```python
from build123d import *

# Parameters (mm, degrees)
SKETCH1_W                  = 480
SKETCH1_H                  = 70
SKETCH1_R                  = 19.15
SKETCH1_R_2                = 2.1
SKETCH1_R_3                = 7.1
BOSS_EXTRUDE1_DEPTH        = 10
M5_TAPPED_HOLE1_D          = 4.2
M5_TAPPED_HOLE1_DEPTH      = 12.4
M5_TAPPED_HOLE1_TIP        = 1.2618073
M5_TAPPED_HOLE2_D          = 4.2
M5_TAPPED_HOLE2_DEPTH      = 12.4
M5_TAPPED_HOLE2_TIP        = 1.2618073
F_3_3_3_3_DIAMETER_HOLE1_D = 3.3


with BuildPart() as part:
    # Sketch1 → Boss-Extrude1 (new body)
    with BuildSketch(Plane.XY):
        Rectangle(SKETCH1_W, SKETCH1_H)
        with Locations((0, -1)):
            Circle(SKETCH1_R, mode=Mode.SUBTRACT)
        with Locations((-23.55, -24.55)):
            Circle(SKETCH1_R_2, mode=Mode.SUBTRACT)
        with Locations((23.55, -24.55)):
            Circle(SKETCH1_R_2, mode=Mode.SUBTRACT)
        with Locations((23.55, 22.55)):
            Circle(SKETCH1_R_2, mode=Mode.SUBTRACT)
        with Locations((-23.55, 22.55)):
            Circle(SKETCH1_R_2, mode=Mode.SUBTRACT)
        with Locations((-215, -5)):
            Circle(SKETCH1_R_3, mode=Mode.SUBTRACT)
        with Locations((215, -5)):
            Circle(SKETCH1_R_3, mode=Mode.SUBTRACT)
    extrude(amount=BOSS_EXTRUDE1_DEPTH)

    # M5 Tapped Hole1
    with Locations(Plane(origin=(0, 35, 0), x_dir=(1, 0, 0), z_dir=(0, 1, 0))):
        with Locations((220, -5), (-220, -5), (-20, -5), (20, -5)):
            Hole(M5_TAPPED_HOLE1_D / 2, depth=M5_TAPPED_HOLE1_DEPTH)
            with Locations((0, 0, -(M5_TAPPED_HOLE1_DEPTH + M5_TAPPED_HOLE1_TIP / 2))):  # 118° drill point
                Cone(0, M5_TAPPED_HOLE1_D / 2, M5_TAPPED_HOLE1_TIP, mode=Mode.SUBTRACT)

    # M5 Tapped Hole2
    with Locations(Plane(origin=(0, -35, 0), x_dir=(-1, 0, 0), z_dir=(0, -1, 0))):
        with Locations((-220, -5), (220, -5)):
            Hole(M5_TAPPED_HOLE2_D / 2, depth=M5_TAPPED_HOLE2_DEPTH)
            with Locations((0, 0, -(M5_TAPPED_HOLE2_DEPTH + M5_TAPPED_HOLE2_TIP / 2))):  # 118° drill point
                Cone(0, M5_TAPPED_HOLE2_D / 2, M5_TAPPED_HOLE2_TIP, mode=Mode.SUBTRACT)

    # Ø3.3 (3.3) Diameter Hole1 (through all)
    with Locations(Plane.XY.offset(10)):
        with Locations((-200, 23), (-120, 23), (-40, 23), (40, 23), (120, 23), (200, 23)):
            Hole(F_3_3_3_3_DIAMETER_HOLE1_D / 2)


solid = part.part
```
Model file for the job. Use its own axes, mm. Round coordinates to 2 decimals unless told otherwise and drop trailing zeros. Order: outer loops, then holes, each group sorted by start corner. A loop starts at its lowest first (then second) coordinate and runs counter-clockwise, first axis right, second up. Notation, with made-up numbers: (20.5, 76.25) -> (25.5, 76.25) arc R33 ccw to (25.5, 111.25) -> close; hole circle Ø2 at (78.5, -4). An arc over 180 degrees is marked (long way). Use one line per item in the form item = value.
Item 1: Drill centre lines: line 1 (Y direction, x = -23.5, z = 6.5); line 2 (Y direction, x = -200, z = 3.75); line 3 (Z direction, x = -20, y = 30.75). Where is each one in solid material? Low to high.
Returned:
line_1 = -35 to -26.65, -22.45 to 20.45, 24.65 to 35
line_2 = -35 to 21.35, 24.65 to 35
line_3 = 0 to 2.9, 7.1 to 10
Item 2: Flat gauge pins, fed straight in: pin 1 Ø3.5 at (x, z) = (20, 5) entering from +Y; pin 2 Ø3 at (x, y) = (-200, 23) entering from -Z; pin 3 Ø2.5 at (x, z) = (-220, 5) entering from +Y. Where does each tip first touch, or does it go through?
Returned:
pin_1 = 22.39
pin_2 = through
pin_3 = 22.09
Item 3: Cut at A-A, the plane y = -5. Write the cut outline in (x, z).
Returned:
outline = (-240, 0) -> (-222.1, 0) -> (-222.1, 10) -> (-240, 10) -> close; (-207.9, 0) -> (-18.73, 0) -> (-18.73, 10) -> (-207.9, 10) -> close; (18.73, 0) -> (207.9, 0) -> (207.9, 10) -> (18.73, 10) -> close; (222.1, 0) -> (240, 0) -> (240, 10) -> (222.1, 10) -> close
Item 4: Pull direction X, two halves, no side cores. Call faces 1 (the face through (-3, 24, 0)), 2 (the face through (221.772, -2.867, 4.93)), 3 (the face through (240, 0, 5)): released by +X, released by -X, zero draft, split by the parting line, or undercut.
Returned:
face_1 = zero draft
face_2 = undercut
face_3 = released by +X
